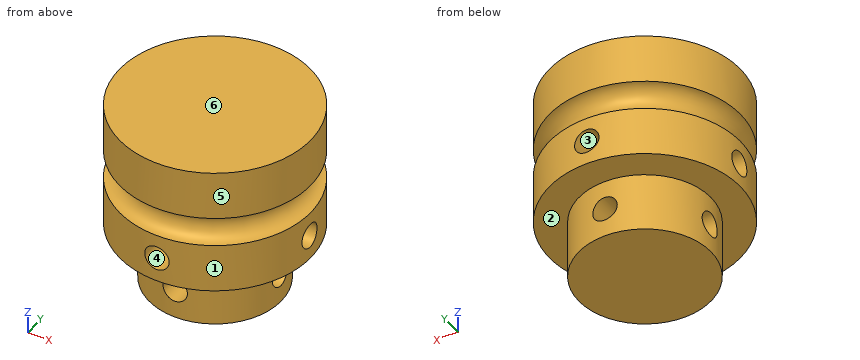
```python
from build123d import *

# Parameters (mm, degrees)
ESBO_O2_R                = 9.75
RESSALTO_EXTRUS_O1_DEPTH = 13
ESBO_O3_R                = 1.5
ESBO_O4_R                = 6.75
RESSALTO_EXTRUS_O2_DEPTH = 6
PADR_OCIRCULAR1_COUNT    = 4
PADR_OCIRCULAR2_COUNT    = 4


with BuildPart() as part:
    # Esboço2 → Ressalto-extrusão1 (new body)
    with BuildSketch(Plane.XY):
        with Locations(Location((0, 0, 0), (0, 0, 180))):
            Circle(ESBO_O2_R)
    extrude(amount=RESSALTO_EXTRUS_O1_DEPTH)

    # Esboço3 → Corte-Revolução1 (revolve, cut)
    with BuildSketch(Plane(origin=(0, 0, 0), x_dir=(1, 0, 0), z_dir=(0, 1, 0)), mode=Mode.PRIVATE) as corte_revolu_o1_sk:
        with Locations((9.75, -6.5)):
            Circle(ESBO_O3_R)
    revolve(corte_revolu_o1_sk.sketch.rotate(Axis((0, 0, 0), (0, 0, 1)), 180), axis=Axis((0, 0, 0), (0, 0, 1)), mode=Mode.SUBTRACT)

    # Esboço4 → Ressalto-extrusão2 (add)
    with BuildSketch(Plane(origin=(0, 0, 0), x_dir=(-1, 0, 0), z_dir=(0, 0, -1))):
        Circle(ESBO_O4_R)
    extrude(amount=RESSALTO_EXTRUS_O2_DEPTH)

    # Esboço15 → Broca de rosquear para tarraxa de M36 (revolve, cut)
    with BuildSketch(Plane(origin=(0, 9.75, 2.5), x_dir=(0, 0, 1), z_dir=(1, 0, 0))):
        Polygon((0, 0), (0, 8.751075774), (1.25, 8), (1.25, 0), align=None)
    broca_de_rosquear_para_tarraxa_de_m36 = revolve(axis=Axis((0, 16.1, 2.5), (0, -1, 0)), mode=Mode.SUBTRACT)

    # PadrãoCircular1: Broca de rosquear para tarraxa de M36 ×4 about axis
    padr_ocircular1_axis = Axis((0, 0, 0), (0, 0, 1))
    for i in range(1, PADR_OCIRCULAR1_COUNT):
        add(broca_de_rosquear_para_tarraxa_de_m36.rotate(padr_ocircular1_axis, i * 360 / PADR_OCIRCULAR1_COUNT), mode=Mode.SUBTRACT)

    # Esboço19 → Broca de rosquear para tarraxa de M310 (revolve, cut)
    with BuildSketch(Plane(origin=(0, 6.75, -3), x_dir=(0, 0, 1), z_dir=(1, 0, 0))):
        Polygon((0, 0), (0, 5.751075774), (1.25, 5), (1.25, 0), align=None)
    broca_de_rosquear_para_tarraxa_de_m310 = revolve(axis=Axis((0, 13.1, -3), (0, -1, 0)), mode=Mode.SUBTRACT)

    # PadrãoCircular2: Broca de rosquear para tarraxa de M310 ×4 about axis
    padr_ocircular2_axis = Axis((0, 0, 0), (0, 0, 1))
    for i in range(1, PADR_OCIRCULAR2_COUNT):
        add(broca_de_rosquear_para_tarraxa_de_m310.rotate(padr_ocircular2_axis, i * 360 / PADR_OCIRCULAR2_COUNT), mode=Mode.SUBTRACT)


solid = part.part
```
Part model, mm, in its own coordinate system. Face numbers are marked on the shaded views. A direction names the side the tool comes from. Round coordinates to 2 decimals unless told otherwise and drop trailing zeros. Write each loop counter-clockwise with the first axis right and the second up, starting at its lowest first coordinate (ties: lowest second). Pieces come first, ordered by that corner, then holes. Notation, with made-up numbers: (-26.5, 50) -> (-10.5, 50) arc R21 ccw to (-10.5, 85) -> close; hole circle Ø5 at (75, -16.5). An arc over 180 degrees is marked (long way). Return JSON: item names as keys, results as strings. Group by question number.
Q1. Saw through at A-A on z = 10.25. Write the cut outline in (x, y).
Q2. Pin check, flat tips, straight feed: pin 1 (3 mm diameter, centred on y = 0, z = -3, fed in from +X); pin 2 (1.5 mm diameter, centred on x = 0, z = 2.5, fed in from -Y); pin 3 (5 mm diameter, centred on y = -4.5, z = 5, fed in from +X). Stop position of each tip, or through.
Q3. Saw through at D-D on z = 5.75. Write the cut outline in (x, y).
Q4. Saw through at B-B on y = 3.25. State how many separate pieces and enclosed holes the cut face has, plus the area to 3 significant figures.
Q5. Mould opens along X. For the marked faces 4, 5 and 6 say: pulls with the +X half, pulls with the -X half, needs draft (parallel to the pull), parting line crosses it, or undercut.
Q6. Probe L1, parallel to Z at x = 0, y = -4.75; L2, parallel to Z at x = 0.75, y = -2; L3, parallel to Y at x = -3.25, z = -2.75. List the from-to ranges inside material, lowest first. Write a range as [from, to].
Q7. Which spindle directions (+Z, -Z, +X, -X, +Y, -Y) get a long thin tool onto all of the face, cutting with end or side? Do the marked faces 1, 2 and 3. Say none if no direction does.
Answer:
{
 "1": {"outline": "circle Ø19.5 at (0, 0)"},
 "2": {"pin 1": "x = 6.75", "pin 2": "y = -1.45", "pin 3": "x = 9.54"},
 "3": {"outline": "circle Ø16.9 at (0, 0)"},
 "4": {"separate pieces": "1", "enclosed holes": "2", "area": "293 mm2"},
 "5": {"face 4": "undercut", "face 5": "parting line crosses it", "face 6": "needs draft"},
 "6": {"L1": "[-6, -4.25], [-1.75, 1.25], [3.75, 13]", "L2": "[-6, -4], [-2, 1.5], [3.5, 13]", "L3": "[-5.92, -1.22], [1.22, 5.92]"},
 "7": {"face 1": "+Z, -Z", "face 2": "-Z", "face 3": "+Y"}
}
